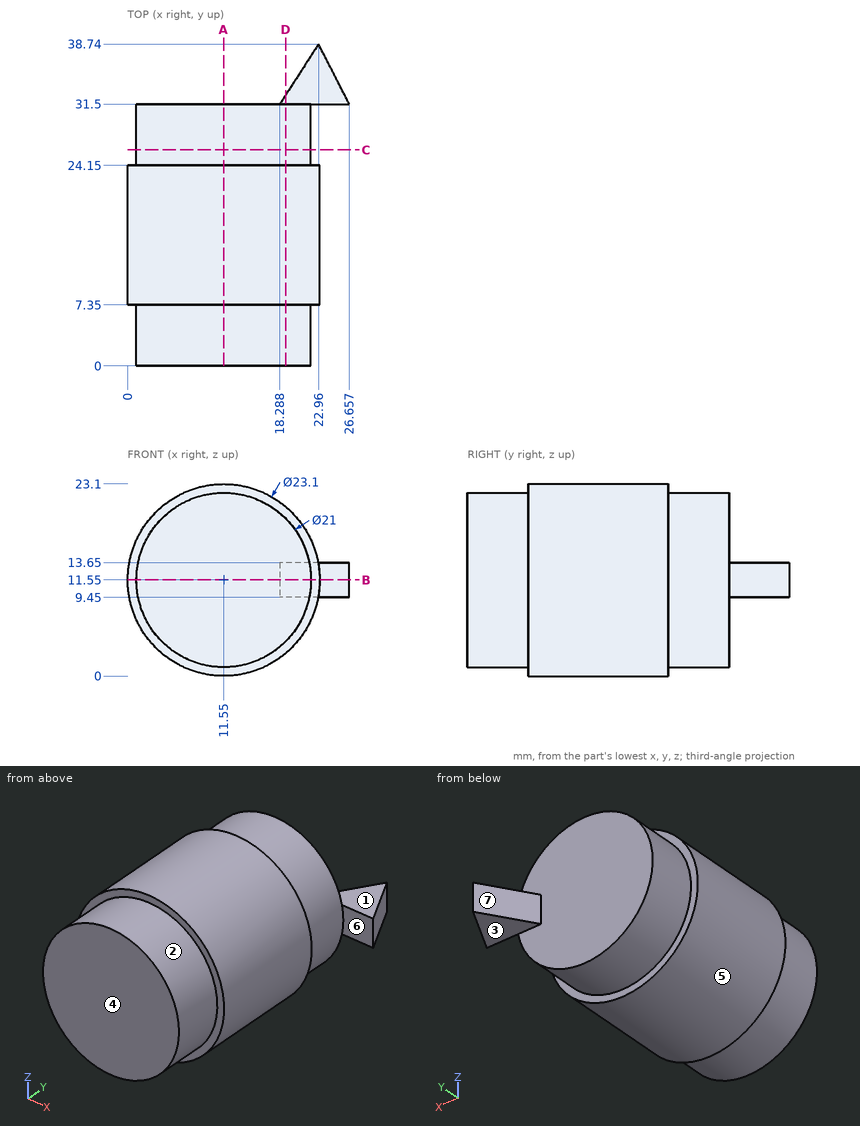
Geometry: see drawing. Coordinates: mm, zero at the bounding-box minimum. A direction names the side the tool comes from. Give positions to 0.01 mm unless a question says otherwise; leave off trailing zeros. Loops run counter-clockwise (first coordinate to the right, second up) from the corner with the lowest first, then second, coordinate; pieces in that order, holes last. Notation, with made-up numbers: (38.5, -32) -> (74.5, -32) arc R18 ccw to (74.5, -3) -> close; hole circle Ø9 at (-5, 47). An arc over 180 degrees is marked (long way). Put each result on its own line as item: value.
1. Cut plane A-A (x = 11.55). Return the cut outline in (y, z).
Taken from the geometry:
outline: (0, 1.05) -> (7.35, 1.05) -> (7.35, 0) -> (24.15, 0) -> (24.15, 1.05) -> (31.5, 1.05) -> (31.5, 22.05) -> (24.15, 22.05) -> (24.15, 23.1) -> (7.35, 23.1) -> (7.35, 22.05) -> (0, 22.05) -> close
2. Cut plane D-D (x = 19). Return the cut outline in (y, z).
Taken from the geometry:
outline: (0, 4.15) -> (7.35, 4.15) -> (7.35, 2.72) -> (24.15, 2.72) -> (24.15, 4.15) -> (31.5, 4.15) -> (31.5, 9.45) -> (32.6, 9.45) -> (32.6, 13.65) -> (31.5, 13.65) -> (31.5, 18.95) -> (24.15, 18.95) -> (24.15, 20.38) -> (7.35, 20.38) -> (7.35, 18.95) -> (0, 18.95) -> close
3. Pull-direction query (Y, two-part tool) for the marked faces 5, 6 and 7; classes: released by +Y, released by -Y, zero draft, split by the parting line, or undercut.
Taken from the geometry:
face 5: zero draft
face 6: undercut
face 7: released by +Y
4. Cut plane B-B (z = 11.55). Return the cut outline in (x, y), plus the area to 3 significant figures.
Taken from the geometry:
outline: (0, 7.35) -> (1.05, 7.35) -> (1.05, 0) -> (22.05, 0) -> (22.05, 7.35) -> (23.1, 7.35) -> (23.1, 24.15) -> (22.05, 24.15) -> (22.05, 31.5) -> (26.66, 31.5) -> (22.96, 38.74) -> (18.29, 31.5) -> (1.05, 31.5) -> (1.05, 24.15) -> (0, 24.15) -> close
area: 727 mm2
5. Set-up query: the marked faces 1, 2, 3 and 4. Return all of +Z, -Z, +X, -X, +Y, -Y with unobstructed straight access to the full face (end or side cutting, diameter ignored); none if empty.
Taken from the geometry:
face 1: +Z, +X, -X, +Y
face 2: -Y
face 3: -Z, +X, -X, +Y
face 4: +Z, -Z, +X, -X, -Y
6. Pin query (flat end, axial travel): P1, Ø2, axis at y = 10, z = 4, coming from the -X side; P2, Ø6, axis at x = 20.5, y = 37, coming from the +Z side; P3, Ø1, axis at x = 8, z = 17, coming from the +Y side. Return the tip coordinate at first contact, or that it passes through.
Taken from the geometry:
P1: stops at x = 2.04
P2: stops at z = 13.65
P3: stops at y = 31.5
7. Cut plane C-C (y = 26). Return the cut outline in (x, z).
Taken from the geometry:
outline: circle Ø21 at (11.55, 11.55)
8. Ray query, line 1 along Y through (x, z) = (18.5, 2.75); line 2 along Z through (x, y) = (12, 2); line 3 along Y through (x, z) = (11.5, 1.5). Return the intervals inside material, ascending. Write a range as [from, to].
Taken from the geometry:
line 1: y = [7.35, 24.15]
line 2: z = [1.06, 22.04]
line 3: y = [0, 31.5]
